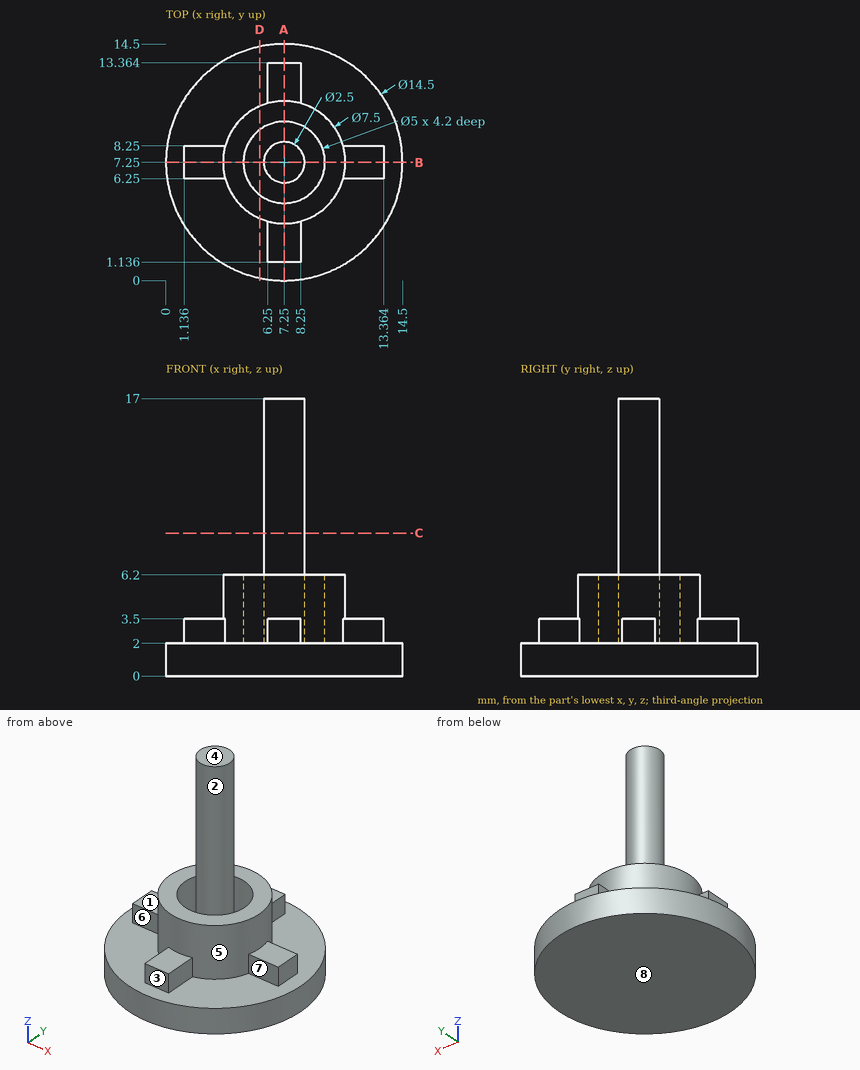
Verification items for this drawing (mm, ordinates from the low corner). A direction names the side the tool comes from. Round coordinates to 2 decimals unless told otherwise and drop trailing zeros. Write each loop counter-clockwise with the first axis right and the second up, starting at its lowest first coordinate (ties: lowest second). Pieces come first, ordered by that corner, then holes. Notation, with made-up numbers: (21.5, -34.5) - (74.5, -34.5) arc R21 cw to (74.5, -8.5) - close; hole circle Ø7 at (10, 64.5). An arc over 180 degrees is marked (long way). Answer as a JSON object with one key per item and string values. Group by question number.
Q1. Section check D-D, the plane x = 5.75. Enter the section's corners in (y, z).
Q2. Tool access check on the marked faces 4, 5, 6, 7 and 8. Record the directions out of +Z, -Z, +X, -X, +Y, -Y that give a thin tool (end or side, any length) a straight path to the whole face; none if there is none.
Q3. Mould release check, pull along Y, two halves, no side actions. Record for the marked faces 1, 2 and 3: released by +Y, released by -Y, zero draft, split by the parting line, or undercut.
Q4. Section check C-C, the plane z = 8.75. Enter the section's corners in (x, y).
Q5. Go/stop test with flat-tipped pins: pin 1 Ø1.2 at (y, z) = (7.5, 3) entering from -X; pin 2 Ø2 at (y, z) = (3.5, 14) entering from +X; pin 3 Ø4 at (x, z) = (3.5, 7.5) entering from -Y (1 decimal); pin 4 Ø1.2 at (y, z) = (3, 3) entering from +X. Record where each tip stops, or that it passes through.
Q6. Section check A-A, the plane x = 7.25. Enter the section's corners in (y, z), plus the area to 3 significant figures.
Q7. Thickness scan on line 1 (Y direction, x = 7.25, z = 4.65); line 2 (Y direction, x = 7.25, z = 3.05); line 3 (Z direction, x = 7.75, y = 11.5). Record the ranges inside material, lowest first.
Found:
{
 "1": {"outline": "(0.16, 0) - (14.34, 0) - (14.34, 2) - (10.69, 2) - (10.69, 6.2) - (9.25, 6.2) - (9.25, 2) - (5.25, 2) - (5.25, 6.2) - (3.81, 6.2) - (3.81, 2) - (0.16, 2) - close"},
 "2": {"face 4": "+Z, +X, -X, +Y, -Y", "face 5": "+Z", "face 6": "+Z, -X, -Y", "face 7": "+Z, +X, -Y", "face 8": "-Z, +X, -X, +Y, -Y"},
 "3": {"face 1": "zero draft", "face 2": "undercut", "face 3": "released by -Y"},
 "4": {"outline": "circle Ø2.5 at (7.25, 7.25)"},
 "5": {"pin 1": "stops at x = 1.14", "pin 2": "passes through", "pin 3": "stops at y = 4.2", "pin 4": "stops at x = 8.25"},
 "6": {"outline": "(0, 0) - (14.5, 0) - (14.5, 2) - (13.36, 2) - (13.36, 3.5) - (11, 3.5) - (11, 6.2) - (9.75, 6.2) - (9.75, 2) - (8.5, 2) - (8.5, 17) - (6, 17) - (6, 2) - (4.75, 2) - (4.75, 6.2) - (3.5, 6.2) - (3.5, 3.5) - (1.14, 3.5) - (1.14, 2) - (0, 2) - close", "area": "84.1 mm^2"},
 "7": {"line 1": "y = 3.5 to 4.75, 6 to 8.5, 9.75 to 11", "line 2": "y = 1.14 to 4.75, 6 to 8.5, 9.75 to 13.36", "line 3": "z = 0 to 3.5"}
}
